The model under review builds one solid part; all positions refer to its coordinate system, in mm. A direction names the side the tool comes from. Round coordinates to 2 decimals unless told otherwise and drop trailing zeros. Loops run counter-clockwise (first coordinate to the right, second up) from the corner with the lowest first, then second, coordinate; pieces in that order, holes last. Notation, with made-up numbers: (-26, 87.5) - (1, 87.5) arc R16 ccw to (1, 102.5) - close; hole circle Ø7 at (7.5, -19.75). An arc over 180 degrees is marked (long way). Answer as CSV lines item,"result".
Autodesk Inventor part; units mm, degrees
ref_plane "YZ Plane" through (0, 0, 0) normal (1, 0, 0) x (0, 1, 0)
ref_plane "XZ Plane" through (0, 0, 0) normal (0, 1, 0) x (-1, 0, 0)
ref_plane "XY Plane" through (0, 0, 0) normal (0, 0, 1) x (1, 0, 0)
sketch "Szkic1" plane through (0, 0, 0) normal (0, 1, 0) x (-1, 0, 0)
  line L0 (-3.5, -2.0207) -> (-3.5, 2.0207)
  line L1 (-3.5, 2.0207) -> (0, 4.0415)
  line L2 (0, 4.0415) -> (3.5, 2.0207)
  line L3 (3.5, 2.0207) -> (3.5, -2.0207)
  line L4 (3.5, -2.0207) -> (0, -4.0415)
  line L5 (0, -4.0415) -> (-3.5, -2.0207)
  point P0 (0, 0)
  point P1 (0, 0)
  dimension "d0" = 7
extrude "Wyciągnięcie proste1" add sketch "Szkic1" along normal blind 40
sketch "Szkic2" plane through (0, 40, 0) normal (0, 1, 0) x (1, 0, 0)
  point P0 (0, 0)
  point P1 (0, 0)
hole "Otwór1" at (0, 40, 0) direction (0, -1, 0) diameter 2.459 depth 8.8 tip angle 118
sketch "Szkic3" plane through (0, 0, 0) normal (0, -1, 0) x (1, 0, 0)
  circle A0 centre (0, 0) radius 1.2295 construction
hole "Otwór2" at (0, 0, 0) direction (0, 1, 0) diameter 2.459 depth 10 tip angle 118
properties part number "CH_01_0021_distans_40mm"
1. Clearance check with flat-ended pins moving along their axes: pin 1 (4 mm diameter, centred on x = 0, z = 0, fed in from -Y); pin 2 (2 mm diameter, centred on x = 0, z = 0, fed in from +Y). State where each tip first meets the part, or that it passes through.
Numbers:
pin 1,"stops at y = 0"
pin 2,"stops at y = 31.06"
2. Tool access review of faces 5 (the face through (0.748, 5.07, 0.976)), 6 (the face through (1.8, 19.7, 3)): name each direction out of +Z, -Z, +X, -X, +Y, -Y from which nothing blocks a thin tool from reaching the whole face with its end or side.
Numbers:
face 5,"-Y"
face 6,"+Z, +X, +Y, -Y"
3. Wall thickness on probe 1 along X at (y, z) = (4.25, 0); probe 2 along Z at (x, y) = (1.25, 14.5); probe 3 along X at (y, z) = (16.5, 2.25): over which ranges is each line inside the solid? List them lowest first.
Numbers:
probe 1,"x = -3.5 to -1.23, 1.23 to 3.5"
probe 2,"z = -3.32 to 3.32"
probe 3,"x = -3.1 to 3.1"
4. Draft analysis for pull direction X (two halves, no side actions). For faces 1 (the face through (-1.726, 19.72, 3.045)), 2 (the face through (3.5, 20, 0)), 3 (the face through (1, 0, 1)), 4 (the face through (0.748, 35.538, -0.976)), state which applies: +X half, -X half, draft (parallel to the pull), parting line (faces both ways), or undercut.
Numbers:
face 1,"-X half"
face 2,"+X half"
face 3,"draft"
face 4,"undercut"
5. Take a section at A-A (y = 7.5). State the section outline as (x, z) points, plus the area to 3 significant figures.
Numbers:
outline,"(-3.5, -2.02) - (0, -4.04) - (3.5, -2.02) - (3.5, 2.02) - (0, 4.04) - (-3.5, 2.02) - close; hole circle Ø2.46 at (0, 0)"
area,"37.7 mm²"
6. Take a section at C-C (x = -2.75). State the section outline as (y, z) points.
Numbers:
outline,"(0, -2.45) - (40, -2.45) - (40, 2.45) - (0, 2.45) - close"
7. Take a section at B-B (z = 3). State the section outline as (x, y) points, plus the area to 3 significant figures.
Numbers:
outline,"(-1.8, 0) - (1.8, 0) - (1.8, 40) - (-1.8, 40) - close"
area,"144 mm²"
